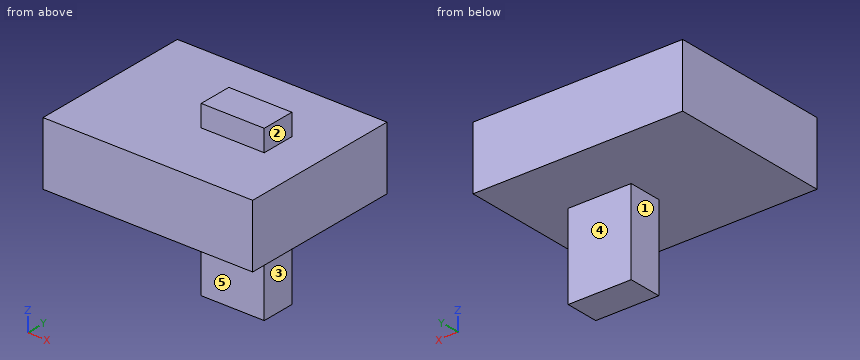
```python
from build123d import *

# Parameters (mm, degrees)
F1_W     = 84.4765
F1_H     = 65.728918
F2_DEPTH = 25.4
F0_W     = 13.509872
F0_H     = 68.137058
F3_DEPTH = 25.4


with BuildPart() as f2:
    # F1 (on Top) → F2 (new body)
    with BuildSketch(Plane.XY):
        Rectangle(F1_W, F1_H)
    extrude(amount=F2_DEPTH)

    # F0 (on Right) → F3 (join)
    with BuildSketch(Plane.YZ):
        Rectangle(F0_W, F0_H)
    extrude(amount=F3_DEPTH)


solid = f2.part
```
Input: part model. Units: mm. Frame: model coordinates. Face numbers are marked on the shaded views. A direction names the side the tool comes from. Give positions to 0.01 mm unless a question says otherwise; leave off trailing zeros. Order: outer loops, then holes, each group sorted by start corner. A loop starts at its lowest first (then second) coordinate and runs counter-clockwise, first axis right, second up.
1. Cut plane A-A (x = 11.5). Return loops of the section in (y, z), and give its area (3 significant figures).
Computed:
outline: (-32.86, 0) - (-6.75, 0) - (-6.75, -34.07) - (6.75, -34.07) - (6.75, 0) - (32.86, 0) - (32.86, 25.4) - (6.75, 25.4) - (6.75, 34.07) - (-6.75, 34.07) - (-6.75, 25.4) - (-32.86, 25.4) - close
area: 2,250 mm2
2. Cut plane C-C (y = -24). Return loops of the section in (x, z), and give its area (3 significant figures).
Computed:
outline: (-42.24, 0) - (42.24, 0) - (42.24, 25.4) - (-42.24, 25.4) - close
area: 2,150 mm2
3. Pin query (flat end, axial travel): pin 1 Ø11 at (y, z) = (2, -25) entering from +X; pin 2 Ø2.5 at (x, z) = (18, 28) entering from +Y; pin 3 Ø1 at (x, y) = (0, 10.5) entering from +Z. Return the tip coordinate at first contact, or that it passes through.
Computed:
pin 1: stops at x = 25.4
pin 2: stops at y = 6.75
pin 3: stops at z = 25.4
4. Line query: probe 1 along Z at (x, y) = (-11, 10.5); probe 2 along Y at (x, z) = (3.5, -9.5). Output: solid intervals per line, ascending.
Computed:
probe 1: z = 0 to 25.4
probe 2: y = -6.75 to 6.75
5. Cut plane B-B (z = 27). Return loops of the section in (x, y), and give its area (3 significant figures).
Computed:
outline: (0, -6.75) - (25.4, -6.75) - (25.4, 6.75) - (0, 6.75) - close
area: 343 mm2
6. Set-up query: the marked faces 1, 2, 3, 4 and 5. Return all of +Z, -Z, +X, -X, +Y, -Y with unobstructed straight access to the full face (end or side cutting, diameter ignored); none if empty.
Computed:
face 1: -Z, -X, +Y, -Y
face 2: +Z, +X, +Y, -Y
face 3: -Z, +X, +Y, -Y
face 4: -Z, +X, -X, +Y
face 5: -Z, +X, -X, -Y
